Read the model definition and answer for the solid it produces. Units are mm, in the model's axes. Face numbers are marked on the shaded views. A direction names the side the tool comes from. Coordinates: 2 decimals unless noted, no trailing zeros. Order: outer loops, then holes, each group sorted by start corner. A loop starts at its lowest first (then second) coordinate and runs counter-clockwise, first axis right, second up.
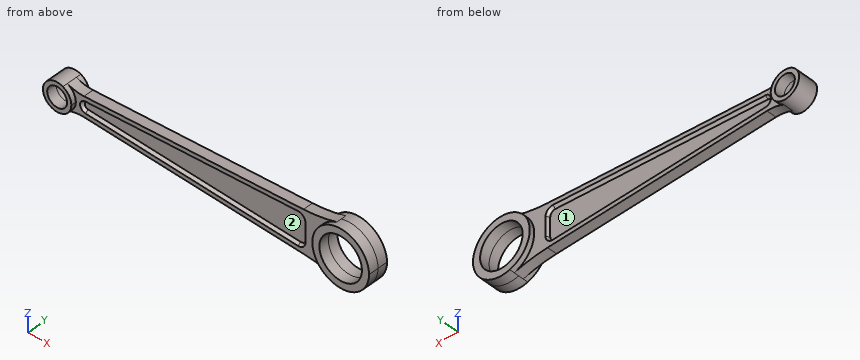
```python
from build123d import *

# Parameters (mm, degrees)
F2_DEPTH = 3.5
F0_R     = 15
F0_R_2   = 7
F3_DEPTH = 7


# Not quite as in the source:
# - a pattern or mirror of a feature is missing from the dataset's text; its kind, count and spacing are read off the source's solid


with BuildPart() as f2:
    # F0 (on Front) → F2 (new body, symmetric)
    with BuildSketch(Plane.XZ):
        with BuildLine():
            ThreePointArc((4.0181641166, 9.157202473), (8.372026074, 5.4689285438), (10, 0))
            ThreePointArc((10, 0), (8.372026074, -5.4689285438), (4.0181641166, -9.157202473))
            ThreePointArc((4.0181641166, -9.157202473), (9.7812118117, -7.3913621026), (15.7960057944, -7))
            Line((15.7960057944, -7), (170.5928896385, -14.9325123484))
            ThreePointArc((170.5928896385, -14.9325123484), (182.467918995, -16.2860219438), (194.0827327125, -19.1046054094))
            ThreePointArc((194.0827327125, -19.1046054094), (180, 0), (194.0827327125, 19.1046054094))
            ThreePointArc((194.0827327125, 19.1046054094), (182.467918995, 16.2860219438), (170.5928896385, 14.9325123484))
            Line((170.5928896385, 14.9325123484), (15.7960057944, 7))
            ThreePointArc((15.7960057944, 7), (9.7812118117, 7.3913621026), (4.0181641166, 9.157202473))
        make_face()
    extrude(amount=F2_DEPTH, both=True)

    # F0 (on Front) → F3 (join, symmetric)
    with BuildSketch(Plane.XZ):
        with BuildLine():
            ThreePointArc((220, 0), (211.86706902, 16.0988407308), (194.0827327125, 19.1046054094))
            ThreePointArc((194.0827327125, 19.1046054094), (180, 0), (194.0827327125, -19.1046054094))
            ThreePointArc((194.0827327125, -19.1046054094), (211.86706902, -16.0988407308), (220, 0))
        make_face()
        with Locations((200, 0)):
            Circle(F0_R, mode=Mode.SUBTRACT)
        with BuildLine():
            ThreePointArc((4.0181641166, -9.157202473), (8.372026074, -5.4689285438), (10, 0))
            ThreePointArc((10, 0), (8.372026074, 5.4689285438), (4.0181641166, 9.157202473))
            ThreePointArc((4.0181641166, 9.157202473), (-10, 0), (4.0181641166, -9.157202473))
        make_face()
        Circle(F0_R_2, mode=Mode.SUBTRACT)
    extrude(amount=F3_DEPTH, both=True)

    # F5 (on offset) → F6 section 0
    with BuildSketch(Plane.XZ.offset(1.5)):
        with BuildLine():
            Line((166.8208787534, 10.1807990679), (16.8720562524, 2.496723933))
            ThreePointArc((16.8720562524, 2.496723933), (14.5, 0), (16.8720562524, -2.496723933))
            Line((16.8720562524, -2.496723933), (166.8208787534, -10.1807990679))
            ThreePointArc((166.8208787534, -10.1807990679), (169.4107131348, -9.2227980591), (170.5, -6.6853855618))
            Line((170.5, -6.6853855618), (170.5, 6.6853855618))
            ThreePointArc((170.5, 6.6853855618), (169.4107131348, 9.2227980591), (166.8208787534, 10.1807990679))
        make_face()
    # F4 (on face) → F6 section 1
    with BuildSketch(Plane.XZ.offset(3.5)):
        with BuildLine():
            Line((166.7441125049, 11.6788334277), (16.7952900039, 3.9947582928))
            ThreePointArc((16.7952900039, 3.9947582928), (13, 0), (16.7952900039, -3.9947582928))
            Line((16.7952900039, -3.9947582928), (166.7441125049, -11.6788334277))
            ThreePointArc((166.7441125049, -11.6788334277), (170.4438759069, -10.3102605579), (172, -6.6853855618))
            Line((172, -6.6853855618), (172, 6.6853855618))
            ThreePointArc((172, 6.6853855618), (170.4438759069, 10.3102605579), (166.7441125049, 11.6788334277))
        make_face()
    f6 = loft(mode=Mode.SUBTRACT)

    # F6_copies: F6 across plane
    add(f6.mirror(Plane.ZX), mode=Mode.SUBTRACT)


solid = f2.part
```
1) A cutting plane is placed at B-B, the plane x = 200. Determine the outline of the cut face in (y, z).
A:
outline: (-7, -20) - (7, -20) - (7, -15) - (-7, -15) - close; (-7, 15) - (7, 15) - (7, 20) - (-7, 20) - close
2) A cutting plane is placed at A-A, the plane x = 0. Determine the outline of the cut face in (y, z), and give its area (3 significant figures).
A:
outline: (-7, -10) - (7, -10) - (7, -7) - (-7, -7) - close; (-7, 7) - (7, 7) - (7, 10) - (-7, 10) - close
area: 84.0 mm2
3) Which of the six approach directions +Z, -Z, +X, -X, +Y, -Y give full straight-line access (tool end or side, diameter ignored) to the marked faces 1 and 2?
A:
face 1: +Y
face 2: -Y
4) Straight lines are drawn through the part: line 1 (Z direction, x = 0, y = -1.5); line 2 (X direction, y = 6.5, z = -4); line 3 (Z direction, x = 200, y = -3.25). For each, find the intervals that lie inside material, in ascending order.
A:
line 1: z = -10 to -7, 7 to 10
line 2: x = -9.17 to -5.74, 5.74 to 9.17, 180.4 to 185.54, 214.46 to 219.6
line 3: z = -20 to -15, 15 to 20
5) Flat-ended cylindrical pins translate along their axes: pin 1 Ø4 at (y, z) = (-4.5, 15) entering from +X; pin 2 Ø11.5 at (x, z) = (86, -9.5) entering from +Y; pin 3 Ø16.5 at (x, z) = (115, -0.5) entering from -Y; pin 4 Ø16 at (x, z) = (0, 0) entering from +Y. Find the tip coordinate at first contact, or state that the pin passes through.
A:
pin 1: stops at x = 215.2
pin 2: stops at y = 3.5
pin 3: stops at y = -3.15
pin 4: stops at y = 7
